Verification items for the finished model (mm, model axes). A direction names the side the tool comes from. Round coordinates to 2 decimals unless told otherwise and drop trailing zeros. Write each loop counter-clockwise with the first axis right and the second up, starting at its lowest first coordinate (ties: lowest second). Pieces come first, ordered by that corner, then holes. Notation, with made-up numbers: M 21.5,42.25 L 46.5,42.25 A23 ccw 46.5,64.25 Z; hole C 81,-5.75 d10. An arc over 180 degrees is marked long. One line per item, written item: value. Start each with the question number.
Item 1: Draft check along Y on faces 5 (the face through (11, -127, 12)), 6 (the face through (4.8, -539.2, -160.4)), 7 (the face through (74.311, -47, -111)), 8 (the face through (-9.271, -343, 0)). Enter one of: +Y half, -Y half, draft (parallel to the pull), parting line (faces both ways), or undercut.
Item 2: Gauge pin test, flat ends, axial feed: pin 1 (1.5 mm diameter, centred on x = -157, y = -345, fed in from -Z); pin 2 (3.5 mm diameter, centred on x = 13.5, z = 5, fed in from -Y); pin 3 (2.5 mm diameter, centred on x = 3, z = 23, fed in from +Y); pin 4 (20.5 mm diameter, centred on y = 29.5, z = -8, fed in from -X). Record the tip position at first contact, or that the pin passes through.
Item 3: Section check C-C, the plane y = -42.5. Record the cut outline in (x, z).
Item 4: Thickness scan on probe 1 along Z at (x, y) = (-28, -217.5); probe 2 along Y at (x, z) = (-37.5, 88.5); probe 3 along Y at (x, z) = (30, -94.5). Record the ranges inside material, lowest first. Write a range as from..to.
Item 5: Section check A-A, the plane x = 41. Record the cut outline in (y, z).
Item 6: Tool access check on faces 1 (the face through (14.81, 25, 4)), 2 (the face through (-105.922, -372, 7)), 3 (the face through (9.271, -343, 0)), 4 (the face through (-3.441, -227.178, -15.497)). Record the directions out of +Z, -Z, +X, -X, +Y, -Y that give a thin tool (end or side, any length) a straight path to the whole face; none if there is none.
Item 7: Section check D-D, the plane x = 0. Record the cut outline in (y, z) (3 decimals), then the cut area to 3 significant figures.
Item 8: Section check B-B, the plane z = 63. Record the cut outline in (x, y), then the cut area to 3 significant figures.
from build123d import *

# Parameters (mm, degrees)
F0_R         = 25.4
F1_DEPTH     = 127
F2_R         = 15.875
F3_DEPTH     = 203.2
F4_W         = 18.542
F4_H         = 25.7731786165
F5_DEPTH     = 25.4
F6_SIZE      = 25.39999
F7_W         = 18.542
F7_H         = 35.9210244843
F8_DEPTH     = 12.7
F9_W         = 29.620467016
F9_H         = 41.2706667472
F10_DEPTH    = 76.2
F11_T1_DEPTH = 290.9034585933
F12_W        = 224.6891856194
F12_H        = 479.333948344
F13_DEPTH    = 25.4
F14_W        = 338.9952555299
F14_H        = 851.445376873
F15_DEPTH    = 25.4


# Not quite as in the source:
# - a fillet or chamfer that OpenCascade refuses, or shapes differently, is made with other operations: its cross-section is extruded or revolved along the edge and cut away or added
# - a fillet or chamfer is up to 0.001 mm smaller than in the source, because OpenCascade refuses the exact size


with BuildPart() as f1:
    # F0 (on Front) → F1 (new body)
    with BuildSketch(Plane.XZ):
        Circle(F0_R)
    extrude(amount=F1_DEPTH)

    # F2 (on face) → F3 (join)
    with BuildSketch(Plane.XZ.offset(127)):
        Circle(F2_R)
    extrude(amount=F3_DEPTH)

    # F4 (on face) → F5 (join)
    with BuildSketch(Plane.XZ.offset(330.2)):
        Rectangle(F4_W, F4_H)
    extrude(amount=F5_DEPTH)

    # F6 (size 25.4 in the source; OpenCascade refuses exactly that, so slightly less here)
    f6_edges = [f1.edges().sort_by_distance(p)[0] for p in [
        (0, -355.6, 12.886589),
    ]]
    chamfer(f6_edges, length=F6_SIZE)

    # F7 (on face) → F8 (join)
    with BuildSketch(Plane(origin=(0, -171.5432946541, 171.5432946541), x_dir=(1, 0, 0), z_dir=(0, -0.7071067812, 0.7071067812))):
        with Locations((0, -242.3349767037)):
            Rectangle(F7_W, F7_H)
    extrude(amount=F8_DEPTH)

    # F9 (on face) → F10 (join)
    with BuildSketch(Plane(origin=(0, 0, 0), x_dir=(-1, 0, 0), z_dir=(0, 1, 0))):
        with Locations((-1.508e-06, -1.0823e-06)):
            Rectangle(F9_W, F9_H)
    extrude(amount=F10_DEPTH)

    # F11: chamfer of 50.8 on 1 edges, made by hand

    # F11_s2 → F11_t1 (cut)
    with BuildSketch(Plane.YZ.offset(-145.4517277887)):
        Polygon((25.4, -20.6353344559), (76.2, 30.1646655441), (76.2, -20.6353344559), align=None)
    extrude(amount=F11_T1_DEPTH, mode=Mode.SUBTRACT)

    # F12 (on face) → F13 (join)
    with BuildSketch(Plane(origin=(0, -180.5235507752, 180.5235507752), x_dir=(1, 0, 0), z_dir=(0, -0.7071067812, 0.7071067812))):
        with Locations((6.4224079251, -255.024516955)):
            Rectangle(F12_W, F12_H)
    extrude(amount=F13_DEPTH)

    # F14 (on face) → F15 (join)
    with BuildSketch(Plane(origin=(0, 23.0176672279, -23.0176672279), x_dir=(1, 0, 0), z_dir=(0, 0.7071067812, -0.7071067812))):
        with Locations((-95.1869599521, 118.0603802204)):
            Rectangle(F14_W, F14_H)
    extrude(amount=F15_DEPTH)


solid = f1.part
Response values:
1. face 5: undercut
1. face 6: -Y half
1. face 7: draft
1. face 8: undercut
2. pin 1: stops at z = -424.78
2. pin 2: stops at y = -393.72
2. pin 3: stops at y = 106.21
2. pin 4: stops at x = -264.68
3. outline: M -264.68,-124.46 L 74.31,-124.46 L 74.31,-88.54 L -264.68,-88.54 Z; C 0,0 d50.8
4. probe 1: z = -299.46..-263.54, 143.55..179.47
4. probe 2: y = -308.47..-272.55, 134.54..170.46
4. probe 3: y = -491.47..-455.55, -48.46..-12.54
5. outline: M -548.28,-151.32 L -530.32,-169.28 L -191.38,169.66 L -209.34,187.62 Z; M -361.5,-407.53 L -343.53,-425.49 L 258.53,176.57 L 240.57,194.53 Z
6. face 1: +Z, +X
6. face 2: +Z, -X, -Y
6. face 3: +X
6. face 4: none
7. outline: M -548.284,-151.316 L -530.323,-169.276 L -364.58,-3.533 L -355.6,-12.513 L -355.6,-12.887 L -330.2,-12.887 L -330.2,-15.875 L -127,-15.875 L -127,-25.4 L 0,-25.4 L 0,-20.635 L 25.4,-20.635 L -361.495,-407.53 L -343.535,-425.491 L 258.528,176.572 L 240.568,194.532 L 66.671,20.635 L 0,20.635 L 0,25.4 L -127,25.4 L -127,15.875 L -330.2,15.875 L -330.2,12.887 L -339.18,21.867 L -191.383,169.664 L -209.343,187.625 Z
7. area: 49,400 mm2
8. outline: M -264.68,109.04 L 74.31,109.04 L 74.31,144.96 L -264.68,144.96 Z; M -105.92,-333.97 L 118.77,-333.97 L 118.77,-298.05 L -105.92,-298.05 Z
8. area: 20,200 mm2
